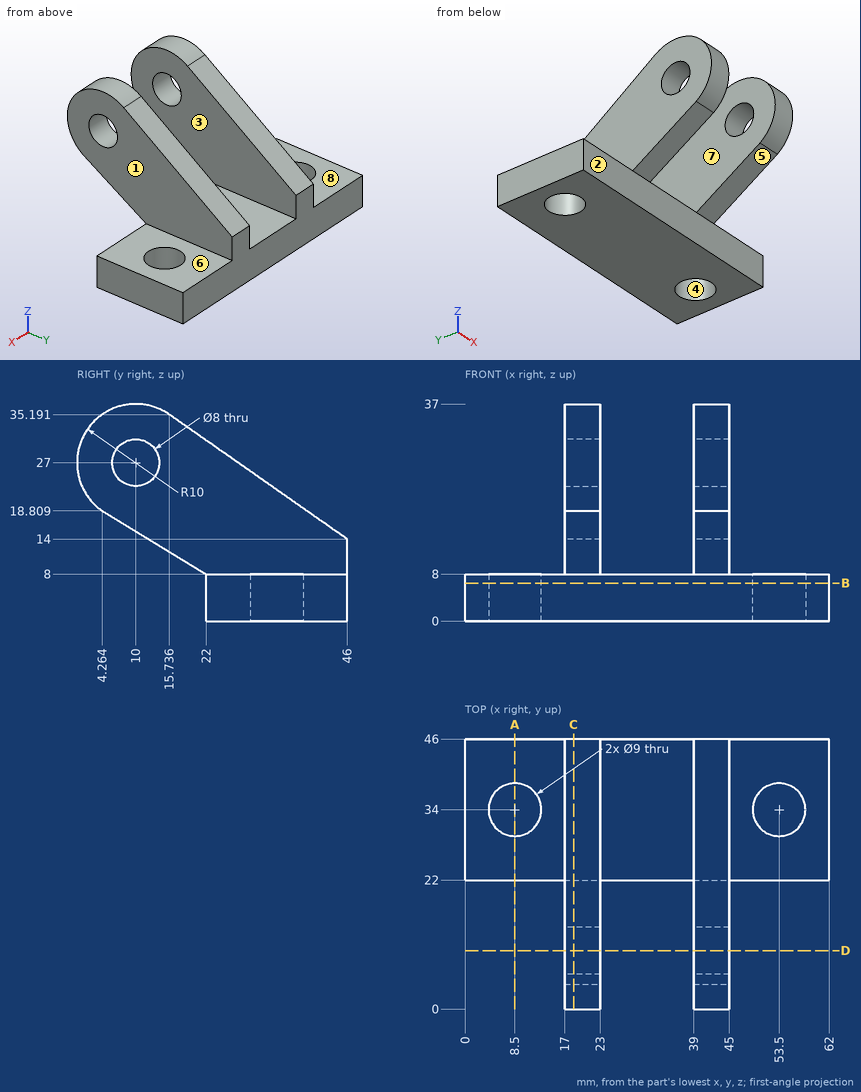
Verification items for this drawing (mm, ordinates from the low corner). A direction names the side the tool comes from. Give positions to 0.01 mm unless a question says otherwise; leave off trailing zeros. Order: outer loops, then holes, each group sorted by start corner. A loop starts at its lowest first (then second) coordinate and runs counter-clockwise, first axis right, second up.
1) Cross-section at C-C (x = 18.5). Record the boundary of the cut face in (y, z) (1 decimal), then the cut area to 3 significant figures.
Results are:
outline: (4.3, 18.8) - (22, 8) - (22, 0) - (46, 0) - (46, 14) - (15.7, 35.2) arc R10 ccw to start; hole circle Ø8 at (10, 27)
area: 923 mm2
2) Cross-section at A-A (x = 8.5). Record the boundary of the cut face in (y, z), then the cut area to 3 significant figures.
Results are:
outline: (22, 0) - (29.5, 0) - (29.5, 8) - (22, 8) - close; (38.5, 0) - (46, 0) - (46, 8) - (38.5, 8) - close
area: 120 mm2
3) Gauge pin test, flat ends, axial feed: pin 1 (3 mm diameter, centred on x = 17.5, z = 13, fed in from -Y) (1 decimal); pin 2 (12 mm diameter, centred on y = 40, z = 19.5, fed in from +X); pin 3 (5 mm diameter, centred on x = 50, y = 36, fed in from +Z); pin 4 (7 mm diameter, centred on x = 53.5, y = 34, fed in from -Z). Record the tip position at first contact, or that the pin passes through.
Results are:
pin 1: stops at y = 11.3
pin 2: stops at x = 45
pin 3: stops at z = 8
pin 4: passes through
4) Cross-section at B-B (z = 6.5). Record the boundary of the cut face in (x, y), then the cut area to 3 significant figures.
Results are:
outline: (0, 22) - (62, 22) - (62, 46) - (0, 46) - close; hole circle Ø9 at (8.5, 34); hole circle Ø9 at (53.5, 34)
area: 1,360 mm2
5) Draft check along X on the marked faces 1, 2 and 3. Enter one of: released by +X, released by -X, zero draft, split by the parting line, or undercut.
Results are:
face 1: released by +X
face 2: zero draft
face 3: undercut
6) Material ranges on probe 1 along X at (y, z) = (10.5, 31.5); probe 2 along Z at (x, y) = (27, 26.5); probe 3 along Y at (x, z) = (48, 2), recorded low to high.
Results are:
probe 1: x = 17 to 23, 39 to 45
probe 2: z = 0 to 8
probe 3: y = 22 to 46
7) Tool access check on the marked faces 4, 5, 6, 7 and 8. Record the directions out of +Z, -Z, +X, -X, +Y, -Y that give a thin tool (end or side, any length) a straight path to the whole face; none if there is none.
Results are:
face 4: +Z, -Z
face 5: -Z, +X, -X, -Y
face 6: +Z, +X, +Y, -Y
face 7: +Z, +Y, -Y
face 8: +Z, -X, +Y, -Y
8) Cross-section at D-D (y = 10). Record the boundary of the cut face in (x, z).
Results are:
outline: (17, 15.31) - (23, 15.31) - (23, 23) - (17, 23) - close; (17, 31) - (23, 31) - (23, 37) - (17, 37) - close; (39, 15.31) - (45, 15.31) - (45, 23) - (39, 23) - close; (39, 31) - (45, 31) - (45, 37) - (39, 37) - close
